Build history of the part. All positions in model axes, mm. Round coordinates to 2 decimals unless told otherwise and drop trailing zeros. Write each loop counter-clockwise with the first axis right and the second up, starting at its lowest first coordinate (ties: lowest second). Pieces come first, ordered by that corner, then holes.
1) Saw through at A-A (z = 34). Write the cut outline in (x, y), plus the area to 3 significant figures.
2) Wall check: probe 1 along X at (y, z) = (1.8, 14); probe 2 along X at (y, z) = (0.4, 34); probe 3 along Z at (x, y) = (24, 0.1). Give the ranges that are in metal, low to high.
3) Saw through at B-B (x = 21). Write the cut outline in (y, z), plus the area to 3 significant figures.
4) Saw through at D-D (x = -7.62). Write the cut outline in (y, z), plus the area to 3 significant figures.
5) Flat gauge pins, fed straight in: pin 1 (3.5 mm diameter, centred on x = 25.34, z = 5.68, fed in from +Y); pin 2 (1.5 mm diameter, centred on y = 2.5, z = 24, fed in from -X); pin 3 (1.3 mm diameter, centred on x = -20.5, y = 0.5, fed in from -Z) (3 decimals). Where does each tip first touch, or does it go through?
6) Saw through at C-C (y = 0.4). State how many separate pieces and enclosed holes the cut face has, plus the area to 3 significant figures.
from build123d import *

# Parameters (mm, degrees)
F0_W     = 30.48
F0_H     = 2.54
F1_DEPTH = 44.45
F0_W_2   = 30.9626
F3_DEPTH = 44.45
F4_R     = 1.905
F4_R_2   = 17.4625
F5_DEPTH = 25.4
F2_W     = 19.05
F2_H     = 3.175
F6_DEPTH = 25.4
F7_R     = 1.524


# Not quite as in the source:
# - a feature names something its author has since deleted; it is built from what else it names


with BuildPart() as f1:
    # F0 (on Top) → F1 (new body)
    with BuildSketch(Plane.XY):
        with Locations((-15.24, 1.27)):
            Rectangle(F0_W, F0_H)
    extrude(amount=F1_DEPTH)

    # F0 (on Top) → F3 (join)
    with BuildSketch(Plane.XY):
        with Locations((15.4813, 1.27)):
            Rectangle(F0_W_2, F0_H)
    extrude(amount=F3_DEPTH)

    # F4 (on face) + F2 (on face) → F5 (cut)
    with BuildSketch(Plane.XZ):
        with Locations((-7.62, 38.7731)):
            Circle(F4_R)
        with Locations((-7.62, 5.6769)):
            Circle(F4_R)
        with Locations((25.3365, 38.7731)):
            Circle(F4_R)
        with Locations((25.3365, 5.6769)):
            Circle(F4_R)
        with Locations((8.7884, 22.225)):
            Circle(F4_R_2)
    with BuildSketch(Plane.XZ):
        with BuildLine():
            Line((-22.098, 9.5885), (-22.098, 12.7635))
            ThreePointArc((-22.098, 12.7635), (-23.8252, 14.4907), (-25.5524, 12.7635))
            Line((-25.5524, 12.7635), (-25.5524, 9.5885))
            ThreePointArc((-25.5524, 9.5885), (-23.8252, 7.8613), (-22.098, 9.5885))
        make_face()
        with BuildLine():
            Line((-22.098, 31.6865), (-22.098, 34.8615))
            ThreePointArc((-22.098, 34.8615), (-23.8252, 36.5887), (-25.5524, 34.8615))
            Line((-25.5524, 34.8615), (-25.5524, 31.6865))
            ThreePointArc((-25.5524, 31.6865), (-23.8252, 29.9593), (-22.098, 31.6865))
        make_face()
        with BuildLine():
            Line((-30.48, 29.337), (-30.48, 15.113))
            ThreePointArc((-30.48, 15.113), (-26.3652, 22.225), (-30.48, 29.337))
        make_face()
    extrude(amount=-F5_DEPTH, mode=Mode.SUBTRACT)

    # F2 (on face) → F6 (cut)
    with BuildSketch(Plane.XZ):
        with Locations((-20.955, 42.8625)):
            Rectangle(F2_W, F2_H)
        with Locations((-20.955, 1.5875)):
            Rectangle(F2_W, F2_H)
    extrude(amount=-F6_DEPTH, mode=Mode.SUBTRACT)

    # F7
    f7_edges = [f1.edges().sort_by_distance(p)[0] for p in [
        (-11.43, 1.27, 41.275),
        (-11.43, 1.27, 44.45),
        (-11.43, 1.27, 0),
        (-11.43, 1.27, 3.175),
        (-30.48, 1.27, 3.175),
        (-30.48, 1.27, 29.337),
        (-30.48, 1.27, 15.113),
        (-30.48, 1.27, 41.275),
        (30.9626, 1.27, 0),
        (30.9626, 1.27, 44.45),
    ]]
    fillet(f7_edges, radius=F7_R)


solid = f1.part
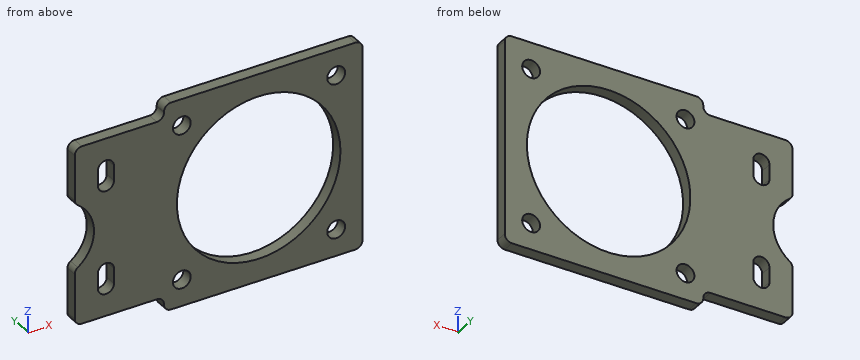
Evaluation:
1. outline: (-30.48, 0) - (-25.55, 0) - (-25.55, 2.54) - (-30.48, 2.54) - close; (-22.1, 0) - (-4.11, 0) - (-4.11, 2.54) - (-22.1, 2.54) - close; (21.68, 0) - (30.96, 0) - (30.96, 2.54) - (21.68, 2.54) - close
1. area: 81.8 mm2
2. probe 1: x = -30.48 to -25.03, -22.62 to -6.62, 24.19 to 30.96
2. probe 2: x = -30.48 to -25.55, -22.1 to -4.11, 21.68 to 30.96
2. probe 3: z = 0 to 4.32, 7.03 to 13.65, 30.8 to 37.42, 40.13 to 44.45
3. outline: (0, 0) - (2.54, 0) - (2.54, 9.74) - (0, 9.74) - close; (0, 34.71) - (2.54, 34.71) - (2.54, 44.45) - (0, 44.45) - close
3. area: 49.5 mm2
4. outline: (0, 0) - (2.54, 0) - (2.54, 3.77) - (0, 3.77) - close; (0, 7.58) - (2.54, 7.58) - (2.54, 16.25) - (0, 16.25) - close; (0, 28.2) - (2.54, 28.2) - (2.54, 36.87) - (0, 36.87) - close; (0, 40.68) - (2.54, 40.68) - (2.54, 44.45) - (0, 44.45) - close
4. area: 63.2 mm2
5. pin 1: passes through
5. pin 2: stops at x = -26.76
5. pin 3: stops at z = 3.175
6. separate pieces: 1
6. enclosed holes: 7
6. area: 1,520 mm2
